```python
from build123d import *

# Parameters (mm, degrees)
SKETCH070_W     = 40.2
SKETCH070_H     = 40.4
PAD024_DEPTH    = 65
SKETCH071_R     = 1.3
POCKET037_DEPTH = 5
PAD025_DEPTH    = 33.5
SKETCH073_R     = 9.05
PAD026_DEPTH    = 11.66
SKETCH074_R     = 2.71
PAD027_DEPTH    = 2.85


with BuildPart() as part:
    # Sketch070 → Pad024 (new body)
    with BuildSketch(Plane.XY):
        Rectangle(SKETCH070_W, SKETCH070_H)
    extrude(amount=PAD024_DEPTH)

    # Sketch071 → Pocket037 (cut)
    with BuildSketch(Plane.XZ.offset(20.2)):
        with Locations((8, 9)):
            Circle(SKETCH071_R)
        with Locations((-8, 9)):
            Circle(SKETCH071_R)
        with Locations((-8, 49)):
            Circle(SKETCH071_R)
        with Locations((8, 49)):
            Circle(SKETCH071_R)
    extrude(amount=-POCKET037_DEPTH, mode=Mode.SUBTRACT)

    # Sketch072 → Pad025 (join)
    with BuildSketch(Plane.XY.offset(65)):
        with BuildLine():
            Line((-17.75, 20.35), (17.75, 20.35))
            ThreePointArc((20.35, 17.75), (19.588478, 19.588478), (17.75, 20.35))
            Line((20.35, 17.75), (20.35, -17.75))
            ThreePointArc((17.75, -20.35), (19.588478, -19.588478), (20.35, -17.75))
            Line((17.75, -20.35), (-17.75, -20.35))
            ThreePointArc((-20.35, -17.75), (-19.588478, -19.588478), (-17.75, -20.35))
            Line((-20.35, -17.75), (-20.35, 17.75))
            ThreePointArc((-17.75, 20.35), (-19.588478, 19.588478), (-20.35, 17.75))
        make_face()
    extrude(amount=PAD025_DEPTH)

    # Sketch073 → Pad026 (join)
    with BuildSketch(Plane.XY):
        Circle(SKETCH073_R)
    extrude(amount=-PAD026_DEPTH)

    # Sketch074 → Pad027 (join)
    with BuildSketch(Plane.XY.offset(98.5)):
        with Locations((-16, 16)):
            Circle(SKETCH074_R)
        with Locations((16, 16)):
            Circle(SKETCH074_R)
        with Locations((16, -16)):
            Circle(SKETCH074_R)
        with Locations((-16, -16)):
            Circle(SKETCH074_R)
    extrude(amount=PAD027_DEPTH)


solid = part.part
```
Design review of the part built by this model. Coordinates are the model's own, in mm. A direction names the side the tool comes from. Coordinates: 2 decimals unless noted, no trailing zeros. Order: outer loops, then holes, each group sorted by start corner. A loop starts at its lowest first (then second) coordinate and runs counter-clockwise, first axis right, second up. Notation, with made-up numbers: M -27.75,8 L 16.25,8 A18 ccw 16.25,30 Z; hole C 2,-2.75 d5. An arc over 180 degrees is marked long. Answer as a JSON object with one key per item and string values. Group by question number.
1) Add section A-A, the plane y = 0. Write out the cut boundary in (x, z).
2) Tool access review of faces 1 (the flat face through (-8, -15.2, 9)), 2 (the flat face through (0, 0, 98.5)), 3 (the cylindrical face through (8.63, 2.72, -5.75)): name each direction out of +Z, -Z, +X, -X, +Y, -Y from which nothing blocks a thin tool from reaching the whole face with its end or side.
3) Wall thickness on L1, parallel to Z at x = -8, y = -18; L2, parallel to Y at x = 15, z = 54; L3, parallel to X at y = 14, z = 6: over which ranges is each line inside the solid? List them lowest first.
4) Mouldability with a two-part tool opening along Y and no side actions: class faces 4 (the flat face through (20.1, 0, 32)), 5 (the cylindrical face through (19.609, 19.568, 81.516)), 6 (the cylindrical face through (-14.75, -18.404, 99.905)) as pulls with the +Y half, pulls with the -Y half, needs draft (parallel to the pull), parting line crosses it, or undercut.
5) Add section B-B, the plane x = 16. Write out the cut boundary in (y, z).
6) Add section D-D, the plane z = 30. Write out the cut boundary in (x, y), then the cut area to 3 significant figures.
7) Add section C-C, the plane y = 16. Write out the cut boundary in (x, z), then the cut area to 3 significant figures.
8) For pin 1 (0.7 mm diameter, centred on x = 19, y = 19.5, fed in from +Z); pin 2 (1.6 mm diameter, centred on x = -8, z = 9, fed in from +Y); pin 3 (1.5 mm diameter, centred on x = 4.5, z = 55, fed in from -Y), all flat-tipped, find the tip position at first contact; note any pin that passes through.
Computed values:
{
 "1": {"outline": "M -20.35,65 L -20.1,65 L -20.1,0 L -9.05,0 L -9.05,-11.66 L 9.05,-11.66 L 9.05,0 L 20.1,0 L 20.1,65 L 20.35,65 L 20.35,98.5 L -20.35,98.5 Z"},
 "2": {"face 1": "-Y", "face 2": "+Z", "face 3": "-Z"},
 "3": {"L1": "z = 0 to 7.7, 10.3 to 47.7, 50.3 to 98.5", "L2": "y = -20.2 to 20.2", "L3": "x = -20.1 to 20.1"},
 "4": {"face 4": "needs draft", "face 5": "pulls with the +Y half", "face 6": "undercut"},
 "5": {"outline": "M -20.35,65 L -20.2,65 L -20.2,0 L 20.2,0 L 20.2,65 L 20.35,65 L 20.35,98.5 L 18.71,98.5 L 18.71,101.35 L 13.29,101.35 L 13.29,98.5 L -13.29,98.5 L -13.29,101.35 L -18.71,101.35 L -18.71,98.5 L -20.35,98.5 Z"},
 "6": {"outline": "M -20.1,-20.2 L 20.1,-20.2 L 20.1,20.2 L -20.1,20.2 Z", "area": "1,620 mm^2"},
 "7": {"outline": "M -20.35,65 L -20.1,65 L -20.1,0 L 20.1,0 L 20.1,65 L 20.35,65 L 20.35,98.5 L 18.71,98.5 L 18.71,101.35 L 13.29,101.35 L 13.29,98.5 L -13.29,98.5 L -13.29,101.35 L -18.71,101.35 L -18.71,98.5 L -20.35,98.5 Z", "area": "4,010 mm^2"},
 "8": {"pin 1": "stops at z = 98.5", "pin 2": "stops at y = 20.2", "pin 3": "stops at y = -20.2"}
}
